Design review of the part shown in the three views and the two pictorial views. Dimensions are in mm from the part's minimum x, y and z. A direction names the side the tool comes from. Coordinates: 2 decimals unless noted, no trailing zeros. Loops run counter-clockwise (first coordinate to the right, second up) from the corner with the lowest first, then second, coordinate; pieces in that order, holes last. Notation, with made-up numbers: (-8, 4.5) - (23, 4.5) arc R11 cw to (23, 23.5) - close; hole circle Ø1 at (-16, 73). An arc over 180 degrees is marked (long way). One line per item, written item: value. Start each with the question number.
1. Insertion check: pin 1 (2 mm diameter, centred on x = 2.5, y = 4.5, fed in from -Z); pin 2 (4 mm diameter, centred on x = 9.5, z = 1.5, fed in from +Y). Each pin has a flat end and moves straight along its axis. Give the tip position at first contact, or say it passes through.
2. Take a section at B-B, the plane x = 2.5. State the section outline as (y, z) points.
3. Take a section at C-C, the plane z = 25.75. State the section outline as (x, y) points.
4. For the marked faces 5 and 6, list the 3-axis set-ups (+Z, -Z, +X, -X, +Y, -Y) from which the entire face can be reached by the end or side of a thin tool; tool diameter is ignored.
5. Take a section at D-D, the plane x = 6.5. State the section outline as (y, z) points.
6. The part is to be moulded in two halves that separate along X. For the marked faces 1, 2, 3 and 4, say which applies: released by +X, released by -X, zero draft, split by the parting line, or undercut.
7. To check wall thickness, follow line 1 (X direction, y = 1, z = 17.5); line 2 (Z direction, x = 9.6, y = 0.5); line 3 (Y direction, x = 2.5, z = 24). State the ranges of each line that lie inside material, in increasing order. Write a range as from..to.
8. Take a section at A-A, the plane y = 4.5. Count the separate pieces of the cut face and the enclosed holes in it, and give its area (3 significant figures).
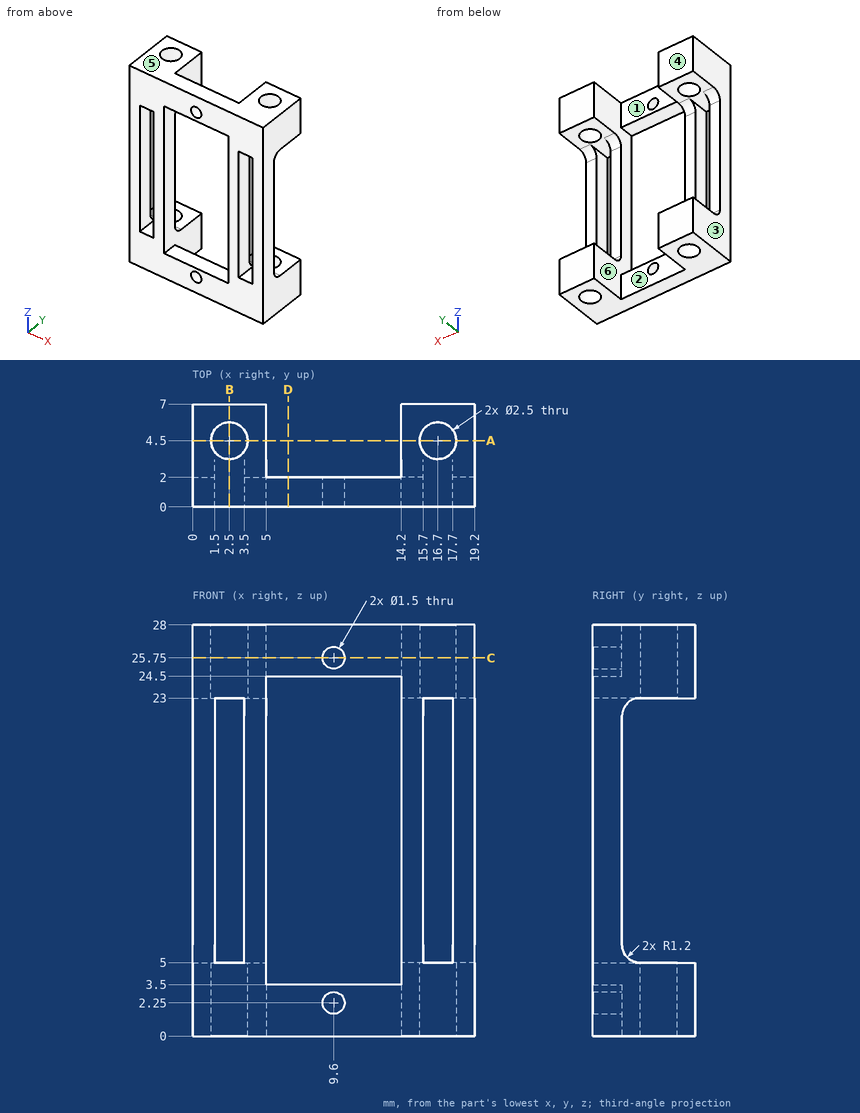
Solutions:
1. pin 1: through
1. pin 2: y = 2
2. outline: (0, 0) - (3.25, 0) - (3.25, 5) - (0, 5) - close; (0, 23) - (3.25, 23) - (3.25, 28) - (0, 28) - close; (5.75, 0) - (7, 0) - (7, 5) - (5.75, 5) - close; (5.75, 23) - (7, 23) - (7, 28) - (5.75, 28) - close
3. outline: (0, 0) - (8.85, 0) - (8.85, 2) - (5, 2) - (5, 7) - (0, 7) - close; (10.35, 0) - (19.2, 0) - (19.2, 7) - (14.2, 7) - (14.2, 2) - (10.35, 2) - close; hole circle Ø2.5 at (2.5, 4.5); hole circle Ø2.5 at (16.7, 4.5)
4. face 5: +Z, +X, -X, +Y, -Y
4. face 6: +Y
5. outline: (0, 0) - (2, 0) - (2, 3.5) - (0, 3.5) - close; (0, 24.5) - (2, 24.5) - (2, 28) - (0, 28) - close
6. face 1: undercut
6. face 2: undercut
6. face 3: released by -X
6. face 4: zero draft
7. line 1: 0..1.5, 3.5..5, 14.2..15.7, 17.7..19.2
7. line 2: 0..1.5, 3..3.5, 24.5..25, 26.5..28
7. line 3: 0..3.25, 5.75..7
8. separate pieces: 8
8. enclosed holes: 0
8. area: 50.0 mm2
